```python
from build123d import *

# Parameters (mm, degrees)
SKETCH_1_R        = 1
EXTRUDE_831_DEPTH = 1.5


with BuildPart() as part:
    # 草图1 → Extrude 831 (new body)
    with BuildSketch(Plane.XY):
        with BuildLine():
            Line((-5.239607816, -3.42469179), (-2.697918198, -6.513350704))
            Line((-2.697918198, -6.513350704), (-4.49653033, -10.855584507))
            ThreePointArc((-4.49653033, -10.855584507), (0, 11.75), (4.49653033, -10.855584507))
            Line((4.49653033, -10.855584507), (2.697918198, -6.513350704))
            Line((2.697918198, -6.513350704), (5.239607816, -3.42469179))
            ThreePointArc((5.239607816, -3.42469179), (8.093813076, -3.84803701), (9.806395304, -1.525802967))
            ThreePointArc((9.806395304, -1.525802967), (0, 9.25), (-9.806395304, -1.525802967))
            ThreePointArc((-9.806395304, -1.525802967), (-8.093813076, -3.84803701), (-5.239607816, -3.42469179))
        make_face()
        with Locations((-5.480027646, -8.003705205)):
            Circle(SKETCH_1_R, mode=Mode.SUBTRACT)
        with Locations(Location((5.480027646, -8.003705205, 0), (0, 0, 180))):
            Circle(SKETCH_1_R, mode=Mode.SUBTRACT)
    extrude(amount=EXTRUDE_831_DEPTH)


solid = part.part
```
Build history of the part. All positions in model axes, mm. A direction names the side the tool comes from. Round coordinates to 2 decimals unless told otherwise and drop trailing zeros. Order: outer loops, then holes, each group sorted by start corner. A loop starts at its lowest first (then second) coordinate and runs counter-clockwise, first axis right, second up. Notation, with made-up numbers: (56.25, -8.5) -> (98.25, -8.5) arc R26 cw to (98.25, 28.5) -> close; hole circle Ø5 at (73, 61.25). An arc over 180 degrees is marked (long way). Answer in a Markdown table with one row per item.
1) Which spindle directions (+Z, -Z, +X, -X, +Y, -Y) get a long thin tool onto all of the face, cutting with end or side? Do faces 1 (the flat face through (5, -4, 0)), 2 (the flat face through (-3.585, -8.654, 0.74)), 3 (the flat face through (-3.987, -4.947, 0.74)). Say none if no direction does.
Values:
| item | result |
|---|---|
| face 1 | -Z, +X, -X, +Y, -Y |
| face 2 | +Z, -Z, -Y |
| face 3 | +Z, -Z |
2) Pin check, flat tip, straight feed: P1, Ø2, axis at x = -5, y = -2, coming from the -Z side. Stop position of the tip, or through.
Values:
| item | result |
|---|---|
| P1 | through |
3) Wall check: L1, parallel to Y at x = 6.25, z = 0.1; L2, parallel to Y at x = 2.75, z = 0.5; L3, parallel to X at y = 7, z = 1.35. Give the ranges that are in metal, low to high.
Values:
| item | result |
|---|---|
| L1 | -9.95 to -8.64, -7.37 to -3.96, 7.01 to 9.95 |
| L2 | -6.64 to -6.45, 8.86 to 11.42 |
| L3 | -9.44 to -6.27, 6.27 to 9.44 |
4) Band-saw the part on A-A on y = 2.5. Give the cut face in (x, z), and give its area (3 significant figures).
Values:
| item | result |
|---|---|
| outline | (-11.48, 0) -> (-9.35, 0) -> (-9.35, 1.5) -> (-11.48, 1.5) -> close; (9.35, 0) -> (11.48, 0) -> (11.48, 1.5) -> (9.35, 1.5) -> close |
| area | 6.39 mm2 |
5) Band-saw the part on B-B on x = -3.25. Give the cut face in (y, z).
Values:
| item | result |
|---|---|
| outline | (-7.85, 0) -> (-5.84, 0) -> (-5.84, 1.5) -> (-7.85, 1.5) -> close; (8.7, 0) -> (11.29, 0) -> (11.29, 1.5) -> (8.7, 1.5) -> close |
6) Band-saw the part on D-D on y = -3.75. Give the cut face in (x, z).
Values:
| item | result |
|---|---|
| outline | (-11.14, 0) -> (-8.3, 0) -> (-8.3, 1.5) -> (-11.14, 1.5) -> close; (-5.73, 0) -> (-4.97, 0) -> (-4.97, 1.5) -> (-5.73, 1.5) -> close; (4.97, 0) -> (5.73, 0) -> (5.73, 1.5) -> (4.97, 1.5) -> close; (8.3, 0) -> (11.14, 0) -> (11.14, 1.5) -> (8.3, 1.5) -> close |
7) Band-saw the part on C-C on z = 1. Give the cut face in (x, y).
Values:
| item | result |
|---|---|
| outline | (-9.81, -1.53) arc R9.85 cw (long way) to (9.81, -1.53) arc R2.8 cw to (5.24, -3.42) -> (2.7, -6.51) -> (4.5, -10.86) arc R11.75 ccw (long way) to (-4.5, -10.86) -> (-2.7, -6.51) -> (-5.24, -3.42) arc R2.8 cw to start; hole circle Ø2 at (-5.48, -8); hole circle Ø2 at (5.48, -8) |
8) Mould opens along X. For faces 4 (the flat face through (5, -4, 1.5)), 5 (the cylindrical face through (-0.45, 11.74, 0.74)), 6 (the cylindrical face through (-8.133, -3.831, 0.74)) say: released by +X, released by -X, zero draft, split by the parting line, or undercut.
Values:
| item | result |
|---|---|
| face 4 | zero draft |
| face 5 | split by the parting line |
| face 6 | undercut |
